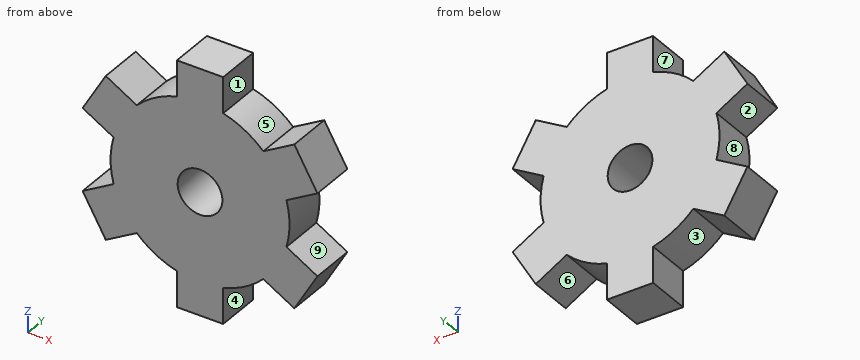
```python
from build123d import *

# Parameters (mm, degrees)
F0_R     = 25.4
F1_DEPTH = 12.7
F3_DEPTH = 12.7
F5_DEPTH = 12.7
F6_COUNT = 6
F7_R     = 6.35
F8_DEPTH = 25.4


with BuildPart() as f1:
    # F0 (on Front) → F1 (new body)
    with BuildSketch(Plane.XZ):
        Circle(F0_R)
    extrude(amount=F1_DEPTH)

    # F2 (on face) → F3 (join)
    with BuildSketch(Plane.XZ.offset(12.7)):
        Polygon((-6.574004, 24.534516), (0, 0), (0, 24.534516), align=None)
        Polygon((0, 24.534516), (0, 0), (6.574004, 24.534516), align=None)
        Polygon((-6.574004, 24.534516), (0, 24.534516), (6.574004, 24.534516), (6.574004, 34.694515), (-6.574004, 34.694515), align=None)
    extrude(amount=-F3_DEPTH)

    # F2 (on face) → F5 (join)
    with BuildSketch(Plane.XZ.offset(12.7)):
        Polygon((-6.574004, 24.534516), (0, 0), (0, 24.534516), align=None)
        Polygon((0, 24.534516), (0, 0), (6.574004, 24.534516), align=None)
        Polygon((-6.574004, 24.534516), (0, 24.534516), (6.574004, 24.534516), (6.574004, 34.694515), (-6.574004, 34.694515), align=None)
    extrude(amount=-F5_DEPTH)

    # F6: F1 ×6 about axis
    f6_axis = Axis((0, -33.893697, 0), (0, 1, 0))


with BuildPart() as f1_1:
    add(f1.part)
    for i in range(1, F6_COUNT):
        add(f1.part.rotate(f6_axis, i * 360 / F6_COUNT))

    # F7 (on face) → F8 (cut)
    with BuildSketch(Plane.XZ.offset(12.7)):
        Circle(F7_R)
    extrude(amount=-F8_DEPTH, mode=Mode.SUBTRACT)


solid = f1_1.part
```
Part model, mm, in its own coordinate system. Face numbers are marked on the shaded views. A direction names the side the tool comes from. Coordinates: 2 decimals unless noted, no trailing zeros. Write each loop counter-clockwise with the first axis right and the second up, starting at its lowest first coordinate (ties: lowest second). Pieces come first, ordered by that corner, then holes.
Item 1: Slice it at C-C (x = 0). Write the cut outline in (y, z), and give its area (3 significant figures).
Item 2: Pin check, flat tips, straight feed: pin 1 (10 mm diameter, centred on x = 5.5, z = 9, fed in from +Y); pin 2 (3 mm diameter, centred on y = -9.5, z = 27.5, fed in from -X); pin 3 (3 mm diameter, centred on y = -4.5, z = 28.5, fed in from +X); pin 4 (2 mm diameter, centred on x = -14.5, y = -6.5, fed in from +Z). Stop position of each tip, or through.
Item 3: Mould opens along Z. For the marked faces 6, 7, 8 and 9 say: released by +Z, released by -Z, zero draft, split by the parting line, or undercut.
Item 4: Slice it at D-D (x = -22). Write the cut outline in (y, z), and give its area (3 significant figures).
Item 5: Which spindle directions (+Z, -Z, +X, -X, +Y, -Y) get a long thin tool onto all of the face, cutting with end or side? Do the marked faces 1, 2, 3, 4 and 5. Say none if no direction does.
Item 6: Slice it at A-A (y = -2). Write the cut outline in (x, z), and give its area (3 significant figures).
Item 7: Probe line 1 (Z direction, x = 0, y = -3); line 2 (Z direction, x = -3.5, y = -5.75); line 3 (X direction, y = -9.5, z = 20). List the from-to ranges inside material, lowest first.
Item 8: Slice it at B-B (z = 0). Write the cut outline in (x, y), and give its area (3 significant figures).
Results found:
1. outline: (-12.7, -34.69) - (0, -34.69) - (0, -6.35) - (-12.7, -6.35) - close; (-12.7, 6.35) - (0, 6.35) - (0, 34.69) - (-12.7, 34.69) - close
1. area: 720 mm2
2. pin 1: stops at y = 0
2. pin 2: stops at x = -6.57
2. pin 3: stops at x = 6.57
2. pin 4: stops at z = 21.52
3. face 6: released by -Z
3. face 7: zero draft
3. face 8: undercut
3. face 9: undercut
4. outline: (-12.7, -20.29) - (0, -20.29) - (0, 20.29) - (-12.7, 20.29) - close
4. area: 515 mm2
5. face 1: +Z, +X, +Y, -Y
5. face 2: -X, +Y, -Y
5. face 3: -Z, +Y, -Y
5. face 4: -Z, +X, +Y, -Y
5. face 5: +Z, +Y, -Y
6. outline: (-33.33, -11.65) - (-26.76, -23.04) - (-17.96, -17.96) arc R25.4 ccw to (-6.57, -24.53) - (-6.57, -34.69) - (6.57, -34.69) - (6.57, -24.53) arc R25.4 ccw to (17.96, -17.96) - (26.76, -23.04) - (33.33, -11.65) - (24.53, -6.57) arc R25.4 ccw to (24.53, 6.57) - (33.33, 11.65) - (26.76, 23.04) - (17.96, 17.96) arc R25.4 ccw to (6.57, 24.53) - (6.57, 34.69) - (-6.57, 34.69) - (-6.57, 24.53) arc R25.4 ccw to (-17.96, 17.96) - (-26.76, 23.04) - (-33.33, 11.65) - (-24.53, 6.57) arc R25.4 ccw to (-24.53, -6.57) - close; hole circle Ø12.7 at (0, 0)
6. area: 2,660 mm2
7. line 1: z = -34.69 to -6.35, 6.35 to 34.69
7. line 2: z = -34.69 to -5.3, 5.3 to 34.69
7. line 3: x = -28.51 to -21.49, -15.66 to 15.66, 21.49 to 28.51
8. outline: (-25.4, -12.7) - (-6.35, -12.7) - (-6.35, 0) - (-25.4, 0) - close; (6.35, -12.7) - (25.4, -12.7) - (25.4, 0) - (6.35, 0) - close
8. area: 484 mm2
